from build123d import *

# Parameters (mm, degrees)
SKETCH1_R               = 12.7
BOSS_EXTRUDE1_DEPTH     = 25.4
SKETCH2_R               = 13.335
BOSS_EXTRUDE2_DEPTH     = 0.508
DRAFT1_ANGLE            = 5
SKETCH5_R               = 14.605
BOSS_EXTRUDE3_DEPTH     = 2.54
CUT_EXTRUDE1_DEPTH      = 36.155380157
CUT_EXTRUDE1_DEPTH_BACK = 36.155380157
SKETCH3_R               = 10.795
SKETCH4_W               = 30.48
SKETCH4_H               = 5.08
SKETCH4_W_2             = 5.08
SKETCH4_H_2             = 30.48
CUT_EXTRUDE2_DEPTH      = 22.86
FILLET3_R               = 0.254


with BuildPart() as part:
    # Sketch1 → Boss-Extrude1 (new body)
    with BuildSketch(Plane(origin=(0, 0, 0), x_dir=(1, 0, 0), z_dir=(0, 1, 0))):
        with Locations(Location((0, 0, 0), (0, 0, 270))):
            Circle(SKETCH1_R)
    extrude(amount=BOSS_EXTRUDE1_DEPTH)

    # Sketch2 → Boss-Extrude2 (add)
    with BuildSketch(Plane(origin=(0, 25.4, 0), x_dir=(1, 0, 0), z_dir=(0, 1, 0))):
        with Locations(Location((0, 0, 0), (0, 0, 270))):
            Circle(SKETCH2_R)
    extrude(amount=BOSS_EXTRUDE2_DEPTH)

    # Draft1
    draft1_faces = [part.faces().sort_by_distance(p)[0] for p in [
        (0, 25.654, -13.335),
    ]]
    draft(draft1_faces, Plane.ZX.offset(25.908), DRAFT1_ANGLE)

    # Sketch5 → Boss-Extrude3 (add)
    with BuildSketch(Plane.XZ):
        with Locations(Location((0, 0, 0), (0, 0, 270))):
            Circle(SKETCH5_R)
    extrude(amount=BOSS_EXTRUDE3_DEPTH)

    # Sketch3 → Cut-Extrude1 (cut, two sides: drawn at the far end of the back side and taken through both)
    with BuildSketch(Plane(origin=(0, 25.908, 0), x_dir=(1, 0, 0), z_dir=(0, 1, 0)).offset(-CUT_EXTRUDE1_DEPTH_BACK)):
        with Locations(Location((0, 0, 0), (0, 0, 270))):
            Circle(SKETCH3_R)
    extrude(amount=CUT_EXTRUDE1_DEPTH + CUT_EXTRUDE1_DEPTH_BACK, mode=Mode.SUBTRACT)

    # Sketch4 → Cut-Extrude2 (cut)
    with BuildSketch(Plane(origin=(0, 25.908, 0), x_dir=(1, 0, 0), z_dir=(0, 1, 0))):
        Rectangle(SKETCH4_W, SKETCH4_H)
        Rectangle(SKETCH4_W_2, SKETCH4_H_2)
    extrude(amount=-CUT_EXTRUDE2_DEPTH, mode=Mode.SUBTRACT)

    # Fillet3
    fillet3_edges = [part.edges().sort_by_distance(p)[0] for p in [
        (-2.54, 25.654219214, -13.113476672),
        (-2.54, 25.654219214, 13.113476672),
        (-9.460695751, 25.4, 9.460695751),
        (-13.113476672, 25.654219214, 2.54),
        (13.113476672, 25.654219214, 2.54),
        (-9.429268927, 25.908, 9.429268927),
        (-9.460695751, 25.4, -9.460695751),
        (-9.429268927, 25.908, -9.429268927),
        (-13.113476672, 25.654219214, -2.54),
        (13.113476672, 25.654219214, -2.54),
        (9.429268927, 25.908, -9.429268927),
        (2.54, 25.654219214, -13.113476672),
        (2.54, 25.654219214, 13.113476672),
        (9.460695751, 25.4, -9.460695751),
        (9.460695751, 25.4, 9.460695751),
        (9.429268927, 25.908, 9.429268927),
    ]]
    fillet(fillet3_edges, radius=FILLET3_R - 0.0001)  # a hair under: the kernel refuses the full size


solid = part.part
Could you check a few things on this model? Use its own coordinates, in mm. A direction names the side the tool comes from. Round coordinates to 2 decimals unless told otherwise and drop trailing zeros. Write each loop counter-clockwise with the first axis right and the second up, starting at its lowest first coordinate (ties: lowest second). Pieces come first, ordered by that corner, then holes. Notation, with made-up numbers: (3, -9) - (9, -9) arc R11 cw to (9, 5) - close; hole circle Ø5 at (-37, 83.25). An arc over 180 degrees is marked (long way). Use a Markdown table: item, result.
Q1. I want a section at A-A (x = 0). List the corners of the cut face in (y, z) for me (3 decimals).
Output values:
| item | result |
|---|---|
| outline | (-2.54, -14.605) - (0, -14.605) - (0, -12.7) - (3.048, -12.7) - (3.048, -10.795) - (-2.54, -10.795) - close; (-2.54, 10.795) - (3.048, 10.795) - (3.048, 12.7) - (0, 12.7) - (0, 14.605) - (-2.54, 14.605) - close |
Q2. I want a section at C-C (y = 5.25). List the corners of the cut face in (x, z) for me (3 decimals).
Output values:
| item | result |
|---|---|
| outline | (-12.443, -2.54) arc R12.7 ccw to (-2.54, -12.443) - (-2.54, -10.492) arc R10.795 cw to (-10.492, -2.54) - close; (-12.443, 2.54) - (-10.492, 2.54) arc R10.795 cw to (-2.54, 10.492) - (-2.54, 12.443) arc R12.7 ccw to start; (2.54, -12.443) arc R12.7 ccw to (12.443, -2.54) - (10.492, -2.54) arc R10.795 cw to (2.54, -10.492) - close; (2.54, 10.492) arc R10.795 cw to (10.492, 2.54) - (12.443, 2.54) arc R12.7 ccw to (2.54, 12.443) - close |
Q3. Thinking about a two-plate mould opening in X: for faces 4 (the cylindrical face through (-4.864, 12.522, 11.732)), 5 (the flat face through (0, 3.048, 12)), 6 (the flat face through (-2.54, 15, -12)), 7 (the flat face through (11, 15, 2.54)), which applies, released by +X, released by -X, zero draft, split by the parting line, or undercut?
Output values:
| item | result |
|---|---|
| face 4 | split by the parting line |
| face 5 | undercut |
| face 6 | undercut |
| face 7 | zero draft |
Q4. For faces 1 (the flat face through (7, 0, 11)), 2 (the flat face through (2.54, 15, -11)), 3 (the flat face through (-12, 3.048, 0)), which set-ups out of +Z, -Z, +X, -X, +Y, -Y let a thin tool reach every point of the face, with its end or its side?
Output values:
| item | result |
|---|---|
| face 1 | none |
| face 2 | +Z, -Z, +Y |
| face 3 | +X, -X, +Y |
Q5. For pin 1 (1.1 mm diameter, centred on x = -1, z = -11.5, fed in from +Y); pin 2 (1.5 mm diameter, centred on y = 8.5, z = 2.5, fed in from -X); pin 3 (1 mm diameter, centred on x = 6.5, y = 8.5, fed in from +Z), each with a flat end and sliding along its axis, tell me the tip position at first contact or that it passes through.
Output values:
| item | result |
|---|---|
| pin 1 | y = 3.05 |
| pin 2 | x = -12.44 |
| pin 3 | z = 11.19 |
Q6. I want a section at B-B (z = 0). List the corners of the cut face in (x, y) for me (3 decimals), plus the area to 3 significant figures.
Output values:
| item | result |
|---|---|
| outline | (-14.605, -2.54) - (-10.795, -2.54) - (-10.795, 3.048) - (-12.7, 3.048) - (-12.7, 0) - (-14.605, 0) - close; (10.795, -2.54) - (14.605, -2.54) - (14.605, 0) - (12.7, 0) - (12.7, 3.048) - (10.795, 3.048) - close |
| area | 31.0 mm2 |
Q7. Please list where these lines run through material, in increasing order: L1, parallel to X at y = 2.5, z = 0 (3 decimals); L2, parallel to Z at x = -8, y = 1; L3, parallel to X at y = 5.5, z = -7.25.
Output values:
| item | result |
|---|---|
| L1 | -12.7 to -10.795, 10.795 to 12.7 |
| L2 | -9.86 to -7.25, 7.25 to 9.86 |
| L3 | -10.43 to -8, 8 to 10.43 |
